```python
from build123d import *

# Parameters (mm, degrees)
SKETCH1_W           = 95.25
SKETCH1_H           = 95.25
BASE_EXTRUDE_DEPTH  = 47.625
SKETCH2_R           = 44.45
BOSS_EXTRUDE1_DEPTH = 355.6
SKETCH3_W           = 95.25
SKETCH3_H           = 95.25
BOSS_EXTRUDE2_DEPTH = 44.45
SKETCH4_R           = 25.4
BOSS_EXTRUDE3_DEPTH = 25.4
CUT_EXTRUDE1_START  = -425.45
SKETCH5_R           = 17.4625
CUT_EXTRUDE1_DEPTH  = 425.45
SKETCH6_R           = 9.525
BOSS_EXTRUDE4_DEPTH = 28.575
SKETCH7_W           = 53.975
SKETCH7_H           = 31.75
CUT_EXTRUDE2_DEPTH  = 485.913042462


with BuildPart() as part:
    # Sketch1 → Base-Extrude (new body)
    with BuildSketch(Plane(origin=(0, 0, 0), x_dir=(0, 0, -1), z_dir=(1, 0, 0))):
        Rectangle(SKETCH1_W, SKETCH1_H)
    extrude(amount=-BASE_EXTRUDE_DEPTH)

    # Sketch2 → Boss-Extrude1 (add)
    with BuildSketch(Plane.ZY.offset(47.625)):
        Circle(SKETCH2_R)
    extrude(amount=BOSS_EXTRUDE1_DEPTH)

    # Sketch3 → Boss-Extrude2 (add)
    with BuildSketch(Plane.ZY.offset(403.225)):
        Rectangle(SKETCH3_W, SKETCH3_H)
    extrude(amount=BOSS_EXTRUDE2_DEPTH)

    # Sketch4 → Boss-Extrude3 (add)
    with BuildSketch(Plane.ZY.offset(447.675)):
        Circle(SKETCH4_R)
    extrude(amount=BOSS_EXTRUDE3_DEPTH)

    # Sketch5 → Cut-Extrude1 (cut)
    with BuildSketch(Plane.ZY.offset(473.075).offset(CUT_EXTRUDE1_START)):
        Circle(SKETCH5_R)
    extrude(amount=CUT_EXTRUDE1_DEPTH, mode=Mode.SUBTRACT)

    # Sketch6 → Boss-Extrude4 (add, symmetric)
    with BuildSketch(Plane.XY):
        with BuildLine():
            Line((38.433186394, 21.19635923), (0, 33.314296353))
            Line((0, 33.314296353), (0, -33.314296353))
            Line((0, -33.314296353), (38.433186394, -21.19635923))
            ThreePointArc((38.433186394, -21.19635923), (53.975, 0), (38.433186394, 21.19635923))
        make_face()
        with Locations((31.75, 0)):
            Circle(SKETCH6_R, mode=Mode.SUBTRACT)
    extrude(amount=BOSS_EXTRUDE4_DEPTH, both=True)

    # Sketch7 → Cut-Extrude2 (cut, through all)
    with BuildSketch(Plane(origin=(0, 47.625, 0), x_dir=(-1, 0, 0), z_dir=(0, 1, 0))):
        with Locations((-26.9875, 0)):
            Rectangle(SKETCH7_W, SKETCH7_H)
    extrude(amount=-CUT_EXTRUDE2_DEPTH, mode=Mode.SUBTRACT)


solid = part.part
```
Source: CAD feature listing. Evaluate the final solid. Frame: model axes, mm. A direction names the side the tool comes from. Round coordinates to 2 decimals unless told otherwise and drop trailing zeros. Loops run counter-clockwise (first coordinate to the right, second up) from the corner with the lowest first, then second, coordinate; pieces in that order, holes last. Notation, with made-up numbers: M 7.5,28 L 27.5,28 A21 cw 27.5,57 Z; hole C -19,33 d6. An arc over 180 degrees is marked long. Use a Markdown table: item, result. Add a question column.
1. Section query A-A on x = 31.75. Return the cut outline in (y, z) (3 decimals), then the cut area to 3 significant figures.
2. Reachability of faces 1 (the flat face through (21, 0, -15.875)), 2 (the flat face through (-23, -47.625, 1)), 3 (the flat face through (21, 0, -28.575)), 4 (the flat face through (-23, 47.625, 1)), 5 (the cylindrical face through (-257.372, -10.626, -13.858)) from +Z, -Z, +X, -X, +Y, -Y: full face, straight path, thin tool, end or side. Return the list, or none.
3. Mould query, pull axis X, two halves, no side actions, for faces 6 (the flat face through (-425, -1, -47.625)), 7 (the flat face through (-47.625, -14, 43)), 8 (the flat face through (0, 1, 1)). Classes: pulls with the +X half, pulls with the -X half, needs draft (parallel to the pull), parting line crosses it, or undercut.
4. Line query: line 1 (X direction, y = -37.5, z = 27.5) (3 decimals); line 2 (X direction, y = 0, z = 21.25) (3 decimals); line 3 (Y direction, x = -336, z = 0). Output: solid intervals per line, ascending.
5. Section query C-C on y = 0. Give the number of separate pieces and of enclosed holes in the cut face, then the cut area to 3 significant figures.
6. Contact query for flat-ended pins moving along their axis: P1, Ø1.5, axis at x = -196.5, y = 16.5, coming from the -Z side; P2, Ø5, axis at x = -178, y = 17.5, coming from the -Z side; P3, Ø25, axis at x = 31.75, y = 0, coming from the -Z side (3 decimals); P4, Ø15, axis at x = 31.75, y = 0, coming from the -Z side. Output: stop coordinate, or through.
Reported:
| question | item | result |
|---|---|---|
| 1 | outline | M -23.304,-28.575 L -9.525,-28.575 L -9.525,-15.875 L -23.304,-15.875 Z; M -23.304,15.875 L -9.525,15.875 L -9.525,28.575 L -23.304,28.575 Z; M 9.525,-28.575 L 23.304,-28.575 L 23.304,-15.875 L 9.525,-15.875 Z; M 9.525,15.875 L 23.304,15.875 L 23.304,28.575 L 9.525,28.575 Z |
| 1 | area | 700 mm² |
| 2 | face 1 | +X, +Y, -Y |
| 2 | face 2 | +Z, -Z, +X, -X, -Y |
| 2 | face 3 | -Z, +X, +Y, -Y |
| 2 | face 4 | +Z, -Z, +X, -X, +Y |
| 2 | face 5 | -X |
| 3 | face 6 | needs draft |
| 3 | face 7 | undercut |
| 3 | face 8 | pulls with the +X half |
| 4 | line 1 | x = -447.675 to -403.225, -47.625 to 0 |
| 4 | line 2 | x = -473.075 to 22.225, 41.275 to 53.975 |
| 4 | line 3 | y = -44.45 to -17.46, 17.46 to 44.45 |
| 5 | separate pieces | 3 |
| 5 | enclosed holes | 0 |
| 5 | area | 27,700 mm² |
| 6 | P1 | stops at z = -41.57 |
| 6 | P2 | stops at z = -41.84 |
| 6 | P3 | stops at z = -28.575 |
| 6 | P4 | passes through |
